Build history of the part. All positions in model axes, mm. Round coordinates to 2 decimals unless told otherwise and drop trailing zeros. Write each loop counter-clockwise with the first axis right and the second up, starting at its lowest first coordinate (ties: lowest second). Pieces come first, ordered by that corner, then holes.
from build123d import *

# Parameters (mm, degrees)
BOSS_EXTRUDE1_DEPTH      = 750
BOSS_EXTRUDE1_DEPTH_BACK = 750


with BuildPart() as part:
    # Sketch1 → Boss-Extrude1 (new, two sides: drawn at the far end of the back side and taken through both)
    with BuildSketch(Plane.XY.offset(-BOSS_EXTRUDE1_DEPTH_BACK)):
        with BuildLine():
            Line((-14, -16), (14, -16))
            ThreePointArc((14, -16), (15.414213562, -15.414213562), (16, -14))
            Line((16, -14), (16, 14))
            ThreePointArc((16, 14), (15.414213562, 15.414213562), (14, 16))
            Line((14, 16), (-14, 16))
            ThreePointArc((-14, 16), (-15.414213562, 15.414213562), (-16, 14))
            Line((-16, 14), (-16, -14))
            ThreePointArc((-16, -14), (-15.414213562, -15.414213562), (-14, -16))
        make_face()
        with BuildLine():
            Line((-14, 14.48), (14, 14.48))
            ThreePointArc((14, 14.48), (14.339411255, 14.339411255), (14.48, 14))
            Line((14.48, 14), (14.48, -14))
            ThreePointArc((14.48, -14), (14.339411255, -14.339411255), (14, -14.48))
            Line((14, -14.48), (-14, -14.48))
            ThreePointArc((-14, -14.48), (-14.339411255, -14.339411255), (-14.48, -14))
            Line((-14.48, -14), (-14.48, 14))
            ThreePointArc((-14.48, 14), (-14.339411255, 14.339411255), (-14, 14.48))
        make_face(mode=Mode.SUBTRACT)
    extrude(amount=BOSS_EXTRUDE1_DEPTH + BOSS_EXTRUDE1_DEPTH_BACK)


solid = part.part
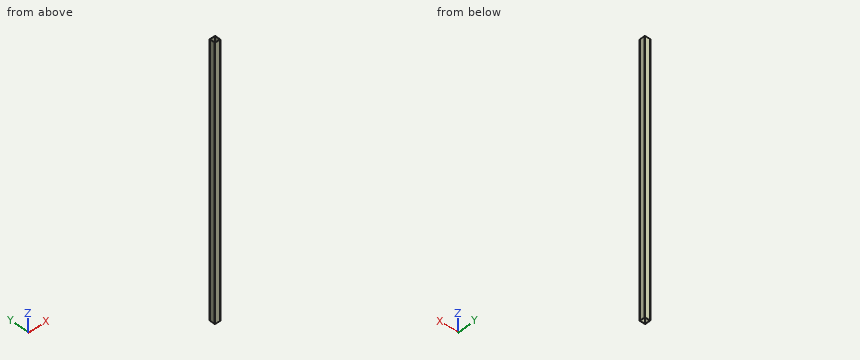
1) Slice it at A-A (y = 5). Write the cut outline in (x, z), plus the area to 3 significant figures.
Results:
outline: (-16, -750) - (-14.48, -750) - (-14.48, 750) - (-16, 750) - close; (14.48, -750) - (16, -750) - (16, 750) - (14.48, 750) - close
area: 4,560 mm2
2) Slice it at C-C (z = 282.5). Write the cut outline in (x, y).
Results:
outline: (-16, -14) arc R2 ccw to (-14, -16) - (14, -16) arc R2 ccw to (16, -14) - (16, 14) arc R2 ccw to (14, 16) - (-14, 16) arc R2 ccw to (-16, 14) - close; hole (-14.48, -14) arc R0.48 ccw to (-14, -14.48) - (14, -14.48) arc R0.48 ccw to (14.48, -14) - (14.48, 14) arc R0.48 ccw to (14, 14.48) - (-14, 14.48) arc R0.48 ccw to (-14.48, 14) - close
3) Wall check: L1, parallel to X at y = 14, z = -279. Give the ranges that are in metal, low to high.
Results:
L1: x = -16 to -14.48, 14.48 to 16
